For this review, take the finished solid that the model builds, in its own axes (mm). Face numbers are marked on the shaded views. A direction names the side the tool comes from. Coordinates: 2 decimals unless noted, no trailing zeros. Order: outer loops, then holes, each group sorted by start corner. A loop starts at its lowest first (then second) coordinate and runs counter-clockwise, first axis right, second up. Notation, with made-up numbers: M 5.5,45.25 L 61.5,45.25 A17 ccw 61.5,56.25 Z; hole C 25.25,-17 d8. An arc over 180 degrees is marked long. Use CSV: the item, a comma, the result in double quotes.
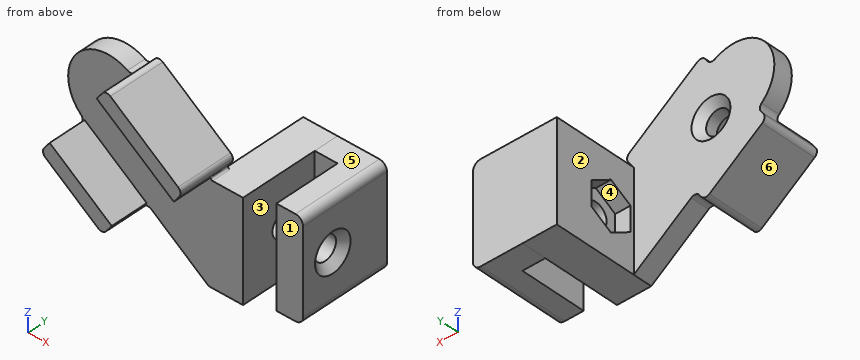
```python
from build123d import *

# Parameters (mm, degrees)
SKETCH_1_R             = 1.55
EXTRUDE_386_DEPTH      = 2.5
EXTRUDE_START          = 2.5
EXTRUDE_629_DEPTH      = 7.5
SKETCH_3_W             = 4.5
SKETCH_3_H             = 12.978713764
EXTRUDE_1_DEPTH        = 13.5
EXTRUDE_START_2        = -0.866441
EXTRUDE_2_DEPTH        = 12.978713764
SKETCH_5_R             = 1.55
CUT_EXTRUDE_1293_DEPTH = 36.225185951
CUT_EXTRUDE_START      = -9
SKETCH_5_3_R           = 1.55
CUT_EXTRUDE_1335_DEPTH = 2
CHAMFER_1_SIZE         = 1
FILLET_5_R             = 0.75
FILLET_6_R             = 0.25
FILLET_8_R             = 1


with BuildPart() as part:
    # 草图1 → Extrude 386 (new body)
    with BuildSketch(Plane(origin=(0, 0, 0), x_dir=(1, 0, 0), z_dir=(0, 1, 0))):
        with BuildLine():
            Line((10.1243866, 13.845154317), (-6.15423406, 2.01804411))
            ThreePointArc((-6.15423406, 2.01804411), (-7.315700706, -5.315167685), (0.017511089, -6.476634331))
            Line((0.017511089, -6.476634331), (10.1243866, 0.866440553))
            Line((10.1243866, 0.866440553), (10.1243866, 13.845154317))
        make_face()
        with Locations(Location((0, 0, 0), (0, 0, 270))):
            Circle(SKETCH_1_R, mode=Mode.SUBTRACT)
    extrude(amount=EXTRUDE_386_DEPTH)

    # 草图2 → Extrude 629 (add)
    with BuildSketch(Plane(origin=(0, 0, 0), x_dir=(1, 0, 0), z_dir=(0, 1, 0)).offset(EXTRUDE_START)):
        Polygon((0.017511089, -6.476634331), (1.193081594, -8.09466832), (11.299957105, -0.751593436), (10.1243866, 0.866440553), align=None)
        Polygon((-7.329804565, 3.636078099), (0.809505765, 9.549633202), (1.98507627, 7.931599213), (-6.15423406, 2.01804411), align=None)
    extrude(amount=-EXTRUDE_629_DEPTH)

    # 草图3 → 限位-1 (add)
    with BuildSketch(Plane(origin=(0, 0, 0), x_dir=(1, 0, 0), z_dir=(0, 1, 0))):
        with Locations((12.3743866, 7.355797435)):
            Rectangle(SKETCH_3_W, SKETCH_3_H)
    extrude(amount=EXTRUDE_1_DEPTH)

    # 草图4 → 限位-2 (add)
    with BuildSketch(Plane.XY.offset(EXTRUDE_START_2)):
        Polygon((14.6243866, 13.5), (21.1243866, 13.5), (21.1243866, 1.5), (17.6243866, 1.5), (17.6243866, 10.25), (14.6243866, 10.25), align=None)
    extrude(amount=-EXTRUDE_2_DEPTH)

    # 草图5 → Cut-Extrude 1293 (cut, through all)
    with BuildSketch(Plane(origin=(21.1243866, 0, 0), x_dir=(0, 0, -1), z_dir=(1, 0, 0))):
        with Locations(Location((7.355797435, 5.75, 0), (0, 0, 90))):
            Circle(SKETCH_5_R)
    extrude(amount=-CUT_EXTRUDE_1293_DEPTH, mode=Mode.SUBTRACT)

    # 草图5<3> → Cut-Extrude 1335 (cut)
    with BuildSketch(Plane(origin=(21.1243866, 0, 0), x_dir=(0, 0, -1), z_dir=(1, 0, 0)).offset(CUT_EXTRUDE_START)):
        Polygon((8.957944432, 2.975), (10.560091429, 5.75), (8.957944432, 8.525), (5.753650438, 8.525), (4.151503441, 5.75), (5.753650438, 2.975), align=None)
        with Locations(Location((7.355797435, 5.75, 0), (0, 0, 90))):
            Circle(SKETCH_5_3_R, mode=Mode.SUBTRACT)
    extrude(amount=-CUT_EXTRUDE_1335_DEPTH, mode=Mode.SUBTRACT)

    # 倒角1
    chamfer_1_edges = [part.edges().sort_by_distance(p)[0] for p in [
        (0, 2.5, -1.55),
        (21.1243866, 4.2, -7.355797435),
    ]]
    chamfer(chamfer_1_edges, length=CHAMFER_1_SIZE)

    # 圆角5
    fillet_5_edges = [part.edges().sort_by_distance(p)[0] for p in [
        (11.299957105, -1.25, 0.751593436),
        (1.193081594, -1.25, 8.09466832),
        (1.98507627, 1.25, -7.931599213),
        (-7.329804565, -1.25, -3.636078099),
        (0.809505765, -1.25, -9.549633202),
        (-6.15423406, 1.25, -2.01804411),
        (0.017511089, 1.25, 6.476634331),
    ]]
    fillet(fillet_5_edges, radius=FILLET_5_R)

    # 圆角6
    fillet_6_edges = [part.edges().sort_by_distance(p)[0] for p in [
        (10.1243866, 1.25, -0.866440553),
    ]]
    fillet(fillet_6_edges, radius=FILLET_6_R)

    # 圆角8
    fillet_8_edges = [part.edges().sort_by_distance(p)[0] for p in [
        (21.1243866, 7.5, -13.845154764),
        (21.1243866, 7.5, -0.866441),
    ]]
    fillet(fillet_8_edges, radius=FILLET_8_R)


solid = part.part
```
Item 1: Add section B-B on x = 13. State the section outline as (y, z) points, and give its area (3 significant figures).
Solutions:
outline,"M 0,-13.85 L 13.5,-13.85 L 13.5,-0.87 L 0,-0.87 Z; hole C 5.75,-7.36 d3.1"
area,"168 mm^2"
Item 2: Add section D-D on x = 16. State the section outline as (y, z) points.
Solutions:
outline,"M 10.25,-13.85 L 13.5,-13.85 L 13.5,-0.87 L 10.25,-0.87 Z"
Item 3: For the marked faces 1, 2 and 3, list the 3-axis set-ups (+Z, -Z, +X, -X, +Y, -Y) from which the entire face can be reached by the end or side of a thin tool; tool diameter is ignored.
Solutions:
face 1,"+Z, -Z, +X, -Y"
face 2,"+Z, -Z, -X, +Y"
face 3,"+Z, -Z, -Y"
Item 4: Add section C-C on z = 3. State the section outline as (x, y) points, and give its area (3 significant figures).
Solutions:
outline,"M -8.26,0 L 4.8,0 L 4.8,-5 L 8.21,-5 L 8.21,2.5 L -8.26,2.5 Z"
area,"58.2 mm^2"
Item 5: Clearance check with flat-ended pins moving along their axes: pin 1 Ø1.9 at (y, z) = (5.75, -7.36) entering from +X; pin 2 Ø2.5 at (x, z) = (15.5, -9.5) entering from -Y; pin 3 Ø6 at (x, y) = (4, 0.5) entering from -Z; pin 4 Ø2 at (x, y) = (13, 5) entering from +Z. State where each tip first meets the part, or that it passes through.
Solutions:
pin 1,"through"
pin 2,"y = 0"
pin 3,"z = -11.58"
pin 4,"z = -0.87"
Item 6: Add section A-A on y = 10.75. State the section outline as (x, z) points.
Solutions:
outline,"M 10.12,-13.85 L 20.12,-13.85 A1 ccw 21.12,-12.85 L 21.12,-1.87 A1 ccw 20.12,-0.87 L 10.12,-0.87 Z"
Item 7: To check wall thickness, follow line 1 along X through (y, z) = (7, -11); line 2 along Z through (x, y) = (12.95, 5.75); line 3 along Y through (x, z) = (-3.75, -1.25). State the ranges of each line that lie inside material, in increasing order. Write a range as [from, to].
Solutions:
line 1,"[10.12, 14.62], [17.62, 21.12]"
line 2,"[-13.85, -8.91], [-5.81, -0.87]"
line 3,"[0, 2.5]"
Item 8: Draft analysis for pull direction Z (two halves, no side actions). For the marked faces 4, 5 and 6, state which applies: released by +Z, released by -Z, zero draft, split by the parting line, or undercut.
Solutions:
face 4,"undercut"
face 5,"released by +Z"
face 6,"released by -Z"
